```python
from build123d import *

# Parameters (mm, degrees)
BOSS_EXTRUDE1_DEPTH = 6


with BuildPart() as part:
    # Sketch1 → Boss-Extrude1 (new body)
    with BuildSketch(Plane(origin=(0, 0, 0), x_dir=(1, 0, 0), z_dir=(0, 1, 0))):
        with BuildLine():
            Line((0, -13.421553628), (101.6, -13.421553628))
            Line((101.6, -13.421553628), (101.6, -70.571553628))
            ThreePointArc((101.6, -70.571553628), (113.157, -82.128553628), (124.714, -70.571553628))
            Line((124.714, -70.571553628), (124.714, 70.571553628))
            ThreePointArc((124.714, 70.571553628), (113.157, 82.128553628), (101.6, 70.571553628))
            Line((101.6, 70.571553628), (101.6, 13.421553628))
            Line((101.6, 13.421553628), (0, 13.421553628))
            Line((0, 13.421553628), (0, -13.421553628))
        make_face()
    extrude(amount=BOSS_EXTRUDE1_DEPTH)

    # Sweep1: sweep along a curve in space
    with BuildLine() as sweep1_path:
        ThreePointArc((113.157, 3, 82.128553628), (104.98496693, 3, 78.743586698), (101.6, 3, 70.571553628))
        Line((101.6, 3, 70.571553628), (101.6, 3, 13.421553628))
        Line((101.6, 3, 13.421553628), (0, 3, 13.421553628))
        Line((0, 3, 13.421553628), (0, 3, -13.421553628))
        Line((0, 3, -13.421553628), (101.6, 3, -13.421553628))
        Line((101.6, 3, -13.421553628), (101.6, 3, -70.571553628))
        ThreePointArc((101.6, 3, -70.571553628), (104.98496693, 3, -78.743586698), (113.157, 3, -82.128553628))
    # Sketch4 → Sweep1 (sweep)
    with BuildSketch(Plane(origin=(113.157, 0, 0), x_dir=(0, 0, -1), z_dir=(1, 0, 0))):
        Polygon((82.128553628, 4.910343042), (82.128553628, 1.060343042), (85.978553628, 2.985343042), align=None)
    sweep(path=sweep1_path.line, transition=Transition.RIGHT)


solid = part.part
```
The model under review builds one solid part; all positions refer to its coordinate system, in mm. A direction names the side the tool comes from. Round coordinates to 2 decimals unless told otherwise and drop trailing zeros. Write each loop counter-clockwise with the first axis right and the second up, starting at its lowest first coordinate (ties: lowest second). Pieces come first, ordered by that corner, then holes.
(1) Wall thickness on L1, parallel to Z at x = 66, y = 0.7; L2, parallel to X at y = 0.3, z = 28.5; L3, parallel to X at y = 4.6, z = -32.5: over which ranges is each line inside the solid? List them lowest first.
(2) We need section A-A on z = -11.5. Give the boundary of the cut face in (x, y), and give its area (3 significant figures).
(3) Insertion check: pin 1 (1.5 mm diameter, centred on y = 2, z = 2.5, fed in from -X); pin 2 (0.5 mm diameter, centred on y = 0.5, z = -50, fed in from -X); pin 3 (0.5 mm diameter, centred on y = 0.5, z = 0.5, fed in from -X). Each pin has a flat end and moves straight along its axis. Give the tip position at first contact, or say it passes through.
(4) Mouldability with a two-part tool opening along Y and no side actions: class faces 4 (the flat face through (99.648, 3.934, 41.597)), 5 (the flat face through (49.6, 2, -15.3)), 6 (the flat face through (113.157, 3, -84)) as +Y half, -Y half, draft (parallel to the pull), parting line (faces both ways), or undercut.
(5) We need section B-B on x = 81. Give the boundary of the cut face in (y, z).
(6) Machinability: for faces 1 (the flat face through (99.7, 2.01, -42.4)), 2 (the flat face through (99.648, 3.934, -42.397)), 3 (the cylindrical face through (116.87, 2.958, 81.516)), which of the approach directions +Z, -Z, +X, -X, +Y, -Y give a long, thin tool a straight path to every point of the face, cutting with its end or side? Answer none if there is none.
(7) We need section C-C on z = -68. Give the boundary of the cut face in (x, y), and give its area (3 significant figures).
Findings below:
1. L1: z = -13.42 to 13.42
1. L2: x = 101.6 to 124.71
1. L3: x = 100.98 to 124.71
2. outline: (-3.85, 2.99) - (0, 1.06) - (0, 0) - (124.71, 0) - (124.71, 6) - (0, 6) - (0, 4.91) - close
2. area: 756 mm2
3. pin 1: stops at x = -3.38
3. pin 2: stops at x = 101.6
3. pin 3: stops at x = 0
4. face 4: +Y half
4. face 5: -Y half
4. face 6: draft
5. outline: (0, -13.42) - (1.06, -13.42) - (2.99, -17.27) - (4.91, -13.42) - (6, -13.42) - (6, 13.42) - (4.91, 13.42) - (2.99, 17.27) - (1.06, 13.42) - (0, 13.42) - close
6. face 1: -Z, -X, -Y
6. face 2: -Z, -X, +Y
6. face 3: +Z
7. outline: (97.75, 2.99) - (101.6, 1.06) - (101.6, 0) - (124.71, 0) - (124.71, 6) - (101.6, 6) - (101.6, 4.91) - close
7. area: 146 mm2
